Autodesk Inventor part; units mm, degrees
ref_plane "YZ Plane" through (0, 0, 0) normal (1, 0, 0) x (0, 1, 0)
ref_plane "XZ Plane" through (0, 0, 0) normal (0, 1, 0) x (-1, 0, 0)
ref_plane "XY Plane" through (0, 0, 0) normal (0, 0, 1) x (1, 0, 0)
sketch "Esquisse2" plane through (0, 0, 0) normal (0, 0, 1) x (1, 0, 0)
  line L0 (-85.4497, 0) -> (85.4497, 0) construction
  line L1 (0, -71.4497) -> (0, 71.4497) construction
  line L2 (-55, -50) -> (55, -50)
  line L3 (60, -45) -> (60, 45)
  line L4 (55, 50) -> (-55, 50)
  line L5 (-60, 45) -> (-60, -45)
  line L6 (-60, -50) -> (60, 50) construction
  line L7 (60, -50) -> (-60, 50) construction
  arc A0 (-55, 50) -> (-60, 45) centre (-55, 45) ccw
  arc A1 (-60, -45) -> (-55, -50) centre (-55, -45) ccw
  arc A2 (55, -50) -> (60, -45) centre (55, -45) ccw
  arc A3 (60, 45) -> (55, 50) centre (55, 45) ccw
  point P0 (0, 0)
  dimension "d0" = 120
  dimension "d1" = 100
  dimension "d2" = 5
extrude "Extrusion1" add sketch "Esquisse2" along normal blind 8
fillet "Congé1" radius 4 8 edges at (58.5355, -48.5355, 8) (60, 0, 8) (58.5355, 48.5355, 8) (0, 50, 8) (-58.5355, 48.5355, 8) (-60, 0, 8) (-58.5355, -48.5355, 8) (0, -50, 8)
sketch "Esquisse3" plane through (0, 0, 8) normal (0, 0, 1) x (1, 0, 0)
  line L0 (-84, 0) -> (84, 0) construction
  line L1 (0, -70) -> (0, 70) construction
  line L2 (55, 50) -> (-55, 50) construction
  line L3 (-60, 45) -> (-60, -45) construction
  line L4 (-60, 50) -> (-26, 50) construction
  line L5 (-26, 50) -> (-26, 30) construction
  line L6 (-26, 30) -> (-60, 30) construction
  line L7 (-60, 30) -> (-60, 50) construction
  line L8 (-26, 30) -> (26.5, 30)
  line L9 (26.5, 30) -> (26.5, -10)
  line L10 (26.5, -10) -> (-26, -10)
  line L11 (-26, -10) -> (-26, 30)
  point P0 (0, 0)
  dimension "d6" = 34
  dimension "d7" = 20
  dimension "d8" = 52.5
  dimension "d9" = 40
extrude "Extrusion2" cut sketch "Esquisse3" against normal through all
properties part number "A2_TopCase" material "Plastique ABS"
Geometry check sheet. Reference: the model listing, model coordinates, mm. A direction names the side the tool comes from. Give positions to 0.01 mm unless a question says otherwise; leave off trailing zeros. Write each loop counter-clockwise with the first axis right and the second up, starting at its lowest first coordinate (ties: lowest second). Pieces come first, ordered by that corner, then holes. Notation, with made-up numbers: (3.5, 89.25) - (26.5, 89.25) arc R10 ccw to (26.5, 107.25) - close; hole circle Ø4 at (26, 32.5). An arc over 180 degrees is marked (long way). Use a Markdown table: item, result.
Q1. Section check B-B, the plane z = 2.5. Enter the section's corners in (x, y).
Computed:
| item | result |
|---|---|
| outline | (-60, -45) arc R5 ccw to (-55, -50) - (55, -50) arc R5 ccw to (60, -45) - (60, 45) arc R5 ccw to (55, 50) - (-55, 50) arc R5 ccw to (-60, 45) - close; hole (-26, -10) - (26.5, -10) - (26.5, 30) - (-26, 30) - close |
Q2. Draft check along X on faces 1 (the face through (26.5, 10, 4)), 2 (the face through (58.797, 0.63, 6.859)), 3 (the face through (-0.8, -10.4, 0)). Enter one of: pulls with the +X half, pulls with the -X half, needs draft (parallel to the pull), parting line crosses it, or undercut.
Computed:
| item | result |
|---|---|
| face 1 | undercut |
| face 2 | pulls with the +X half |
| face 3 | needs draft |
Q3. Section check A-A, the plane x = 1. Enter the section's corners in (y, z), then the cut area to 3 significant figures.
Computed:
| item | result |
|---|---|
| outline | (-50, 0) - (-10, 0) - (-10, 8) - (-46, 8) arc R4 ccw to (-50, 4) - close; (30, 0) - (50, 0) - (50, 4) arc R4 ccw to (46, 8) - (30, 8) - close |
| area | 473 mm² |
Q4. Section check C-C, the plane y = 0. Enter the section's corners in (x, z), then the cut area to 3 significant figures.
Computed:
| item | result |
|---|---|
| outline | (-60, 0) - (-26, 0) - (-26, 8) - (-56, 8) arc R4 ccw to (-60, 4) - close; (26.5, 0) - (60, 0) - (60, 4) arc R4 ccw to (56, 8) - (26.5, 8) - close |
| area | 533 mm² |
Q5. Set-up check for faces 4 (the face through (0, 30, 4)), 5 (the face through (60, -1, 2)): record each of +Z, -Z, +X, -X, +Y, -Y from which the full face is reachable in a straight line by a thin tool's end or side.
Computed:
| item | result |
|---|---|
| face 4 | +Z, -Z |
| face 5 | +Z, -Z, +X, +Y, -Y |
Q6. Thickness scan on L1, parallel to Y at x = 19, z = 3.5; L2, parallel to X at y = 21, z = 4; L3, parallel to Y at x = 19, z = 5.25. Record the ranges inside material, lowest first. Write a range as [from, to].
Computed:
| item | result |
|---|---|
| L1 | y = [-50, -10], [30, 50] |
| L2 | x = [-60, -26], [26.5, 60] |
| L3 | y = [-49.8, -10], [30, 49.8] |
